Geometry: final body of the model. Coordinates: model frame, mm. A direction names the side the tool comes from. Coordinates: 2 decimals unless noted, no trailing zeros. Loops run counter-clockwise (first coordinate to the right, second up) from the corner with the lowest first, then second, coordinate; pieces in that order, holes last. Notation, with made-up numbers: (-33, -28.5) - (10, -28.5) arc R22 ccw to (10, 6.5) - close; hole circle Ø1 at (44, 52.25). An arc over 180 degrees is marked (long way). Put each result on its own line as item: value. Start each with the question number.
1) Contact query for flat-ended pins moving along their axis: pin 1 Ø4.5 at (x, y) = (47, 83.4) entering from -Z; pin 2 Ø1.4 at (y, z) = (2.5, 4.5) entering from +X; pin 3 Ø0.8 at (x, z) = (45.5, 2) entering from -Y; pin 4 Ø1.2 at (x, y) = (26.5, 52) entering from +Z. Output: stop coordinate, or through.
2) Section C-C on x = 35.9. Output: boundary loops of the cut face in (y, z), and give its area (3 significant figures).
3) Section B-B on x = 24.5. Output: boundary loops of the cut face in (y, z).
4) Draft query along X for faces 1 (the cylindrical face through (52.57, 86.9, 2.46)), 2 (the cylindrical face through (3.87, 50.71, 1.98)), 3 (the flat face through (42.9, 54.2, 5)). Return one class per face: +X half, -X half, draft (parallel to the pull), parting line (faces both ways), or undercut.
5) Reachability of faces 4 (the flat face through (52, 28, 4)), 5 (the flat face through (27, 5, 2)) from +Z, -Z, +X, -X, +Y, -Y: full face, straight path, thin tool, end or side. Return the list, or none.
6) Material intervals for line 1 along X through (y, z) = (24, 1.8); line 2 along Y through (x, z) = (34, 2.5); line 3 along X through (y, z) = (7.5, 3.6), sorted ascending. Write a range as from..to.
7) Section A-A on y = 13.5. Output: boundary loops of the cut face in (x, z).
8) Section D-D on z = 1.9. Count the separate pieces of the cut face and the enclosed holes in it, and give its area (3 significant figures).
```python
from build123d import *

# Parameters (mm, degrees)
SKETCH1_R           = 2.9
SKETCH1_R_2         = 1.35
BOSS_EXTRUDE1_DEPTH = 5
CUT_EXTRUDE1_DEPTH  = 5
CUT_EXTRUDE2_DEPTH  = 5
CHAMFER1_SIZE       = 0.4
CHAMFER2_SIZE       = 0.2
FILLET1_R           = 3
FILLET2_R           = 5
SKETCH4_W           = 20.9
SKETCH4_H           = 5
CUT_EXTRUDE3_DEPTH  = 1.7
SKETCH5_W           = 8
SKETCH5_H           = 9.98481564
CUT_EXTRUDE5_DEPTH  = 1.7
CUT_EXTRUDE6_DEPTH  = 1.7


with BuildPart() as part:
    # Sketch1 → Boss-Extrude1 (new body)
    with BuildSketch(Plane.XY):
        with BuildLine():
            Line((0, 0), (54, 0))
            Line((54, 0), (54, 83.4))
            ThreePointArc((54, 83.4), (52.535533906, 86.935533906), (49, 88.4))
            Line((49, 88.4), (5, 88.4))
            ThreePointArc((5, 88.4), (1.464466094, 86.935533906), (0, 83.4))
            Line((0, 83.4), (0, 0))
        make_face()
        with Locations((7, 83.4)):
            Circle(SKETCH1_R, mode=Mode.SUBTRACT)
        with Locations((47, 83.4)):
            Circle(SKETCH1_R, mode=Mode.SUBTRACT)
        with Locations((2.9, 54.7)):
            Circle(SKETCH1_R_2, mode=Mode.SUBTRACT)
        with Locations((51.1, 53.4)):
            Circle(SKETCH1_R_2, mode=Mode.SUBTRACT)
        with Locations((8, 2.6)):
            Circle(SKETCH1_R_2, mode=Mode.SUBTRACT)
        with Locations((35.9, 2.6)):
            Circle(SKETCH1_R_2, mode=Mode.SUBTRACT)
    extrude(amount=BOSS_EXTRUDE1_DEPTH)

    # Sketch2 → Cut-Extrude1 (cut)
    with BuildSketch(Plane.XY.offset(5)):
        Polygon((5.5, 0), (3, 2.5), (0, 2.5), (0, 0), align=None)
        Polygon((38.4, 0), (40.9, 2.5), (54, 2.5), (54, 0), align=None)
    extrude(amount=-CUT_EXTRUDE1_DEPTH, mode=Mode.SUBTRACT)

    # Sketch3 → Cut-Extrude2 (cut)
    with BuildSketch(Plane.XY.offset(5)):
        with BuildLine():
            Line((12, 81), (12, 78.4))
            Line((12, 78.4), (7.4, 78.4))
            ThreePointArc((7.4, 78.4), (3.864466094, 76.935533906), (2.4, 73.4))
            Line((2.4, 73.4), (2.4, 61.96963128))
            ThreePointArc((2.4, 61.96963128), (3.818077427, 58.48110284), (7.267932273, 56.971375773))
            Line((7.267932273, 56.971375773), (46.467932273, 55.935603416))
            ThreePointArc((46.467932273, 55.935603416), (50.088528441, 57.35193635), (51.6, 60.933858923))
            Line((51.6, 60.933858923), (51.6, 73.4))
            ThreePointArc((51.6, 73.4), (50.135533906, 76.935533906), (46.6, 78.4))
            Line((46.6, 78.4), (42, 78.4))
            Line((42, 78.4), (42, 81))
            ThreePointArc((42, 81), (40.535533906, 84.535533906), (37, 86))
            Line((37, 86), (17, 86))
            ThreePointArc((17, 86), (13.464466094, 84.535533906), (12, 81))
        make_face()
        with BuildLine():
            Line((7.532067727, 52.164396584), (46.732067727, 51.128624227))
            ThreePointArc((46.732067727, 51.128624227), (50.181922573, 49.61889716), (51.6, 46.13036872))
            Line((51.6, 46.13036872), (51.6, 10))
            ThreePointArc((51.6, 10), (50.135533906, 6.464466094), (46.6, 5))
            Line((46.6, 5), (7.4, 5))
            ThreePointArc((7.4, 5), (3.864466094, 6.464466094), (2.4, 10))
            Line((2.4, 10), (2.4, 47.166141077))
            ThreePointArc((2.4, 47.166141077), (3.911471559, 50.74806365), (7.532067727, 52.164396584))
        make_face()
    extrude(amount=-CUT_EXTRUDE2_DEPTH, mode=Mode.SUBTRACT)

    # Chamfer1
    chamfer1_edges = [part.edges().sort_by_distance(p)[0] for p in [
        (4.1, 83.4, 0),
        (4.1, 83.4, 5),
        (44.1, 83.4, 0),
        (44.1, 83.4, 5),
    ]]
    chamfer(chamfer1_edges, length=CHAMFER1_SIZE)

    # Chamfer2
    chamfer2_edges = [part.edges().sort_by_distance(p)[0] for p in [
        (1.55, 54.7, 0),
        (1.55, 54.7, 5),
        (49.75, 53.4, 0),
        (49.75, 53.4, 5),
        (6.65, 2.6, 0),
        (6.65, 2.6, 5),
        (34.55, 2.6, 0),
        (34.55, 2.6, 5),
    ]]
    chamfer(chamfer2_edges, length=CHAMFER2_SIZE)

    # Fillet1
    fillet1_edges = [part.edges().sort_by_distance(p)[0] for p in [
        (42, 78.4, 2.5),
        (12, 78.4, 2.5),
    ]]
    fillet(fillet1_edges, radius=FILLET1_R)

    # Fillet2
    # the kernel refuses this fillet: 5 mm, written as the material it takes off along each edge
    with BuildSketch(Plane(origin=(0, 2.5, 16.456439237), x_dir=(0, 1, 0), z_dir=(0, 0, -1))) as fillet2_piece_1:
        with BuildLine():
            CenterArc((4.582575695, 5), FILLET2_R, 203.578178478, 66.421821522)
            Line((0, 3), (-0.091651514, 2.96))
            ThreePointArc((-0.091651514, 2.96), (-0.1, 1.5), (-0.1, 0))
            Line((-0.1, 0), (0, -0.1))
            Line((0, -0.1), (4.582575695, -0.1))
            Line((4.582575695, -0.1), (4.582575695, 0))
        make_face()
    extrude(amount=27.912878475, mode=Mode.SUBTRACT)
    with BuildSketch(Plane(origin=(54, 2.5, 17.5), x_dir=(0, 1, 0), z_dir=(0, 0, -1))) as fillet2_piece_2:
        with BuildLine():
            CenterArc((FILLET2_R, -FILLET2_R), FILLET2_R, 90, 90)
            Line((0, -FILLET2_R), (-FILLET2_R * 0.02, -FILLET2_R))
            Line((-FILLET2_R * 0.02, -FILLET2_R), (-FILLET2_R * 0.02, FILLET2_R * 0.02))
            Line((-FILLET2_R * 0.02, FILLET2_R * 0.02), (FILLET2_R, FILLET2_R * 0.02))
            Line((FILLET2_R, FILLET2_R * 0.02), (FILLET2_R, 0))
        make_face()
    extrude(amount=30, mode=Mode.SUBTRACT)

    # Sketch4 → Cut-Extrude3 (cut)
    with BuildSketch(Plane.XY.offset(5)):
        with Locations((21.95, 2.5)):
            Rectangle(SKETCH4_W, SKETCH4_H)
    extrude(amount=-CUT_EXTRUDE3_DEPTH, mode=Mode.SUBTRACT)

    # Sketch5 → Cut-Extrude5 (cut)
    with BuildSketch(Plane.XY.offset(5)):
        Polygon((2, 51.696310663), (52, 50.375172451), (52, 4.5), (2, 4.5), align=None)
        with Locations((6, 62.69240782)):
            Rectangle(SKETCH5_W, SKETCH5_H)
    extrude(amount=-CUT_EXTRUDE5_DEPTH, mode=Mode.SUBTRACT)

    # Sketch6 → Cut-Extrude6 (cut)
    with BuildSketch(Plane.XY.offset(5)):
        Polygon((48.1, 53.891781634), (5.9, 55.006822285), (5.9, 50.553811317), (48.1, 49.438770667), align=None)
    extrude(amount=-CUT_EXTRUDE6_DEPTH, mode=Mode.SUBTRACT)


solid = part.part
```
Answer block:
1. pin 1: passes through
1. pin 2: stops at x = 51.55
1. pin 3: stops at y = 2.5
1. pin 4: stops at z = 3.3
2. outline: (0, 0) - (1.05, 0) - (1.25, 0.2) - (1.25, 4.8) - (1.05, 5) - (0, 5) - close; (3.95, 0.2) - (4.15, 0) - (5, 0) - (5, 3.3) - (4.5, 3.3) - (4.5, 5) - (4.15, 5) - (3.95, 4.8) - close; (51.41, 0) - (56.21, 0) - (56.21, 5) - (54.21, 5) - (54.21, 3.3) - (51.41, 3.3) - close; (86, 0) - (88.4, 0) - (88.4, 5) - (86, 5) - close
2. area: 41.8 mm²
3. outline: (0, 0) - (5, 0) - (5, 3.3) - (0, 3.3) - close; (51.72, 0) - (56.52, 0) - (56.52, 5) - (54.52, 5) - (54.52, 3.3) - (51.72, 3.3) - close; (86, 0) - (88.4, 0) - (88.4, 5) - (86, 5) - close
4. face 1: +X half
4. face 2: undercut
4. face 3: draft
5. face 4: +Z
5. face 5: +Z, -Z
6. line 1: x = 0..2.4, 51.6..54
6. line 2: y = 0..5, 51.47..56.27, 86..88.4
6. line 3: x = 0..2, 52..54
7. outline: (0, 0) - (2.4, 0) - (2.4, 3.3) - (2, 3.3) - (2, 5) - (0, 5) - close; (51.6, 0) - (54, 0) - (54, 5) - (52, 5) - (52, 3.3) - (51.6, 3.3) - close
8. separate pieces: 1
8. enclosed holes: 8
8. area: 1,080 mm²
